Here's how the part is built. I have some questions about the finished solid (model axes, mm). A direction names the side the tool comes from. Round coordinates to 2 decimals unless told otherwise and drop trailing zeros. Write each loop counter-clockwise with the first axis right and the second up, starting at its lowest first coordinate (ties: lowest second). Pieces come first, ordered by that corner, then holes. Notation, with made-up numbers: (-34, 59) -> (-6, 59) arc R29 cw to (-6, 97) -> close; hole circle Ø5 at (19.5, 77.5). An arc over 180 degrees is marked (long way). Answer as CSV lines item,"result".
from build123d import *

# Parameters (mm, degrees)
EXTRUDE_1_DEPTH = 2
EXTRUDE_2_DEPTH = 1


with BuildPart() as part:
    # Эскиз1 → Бобышка-Вытянуть1 (new body)
    with BuildSketch(Plane.XY):
        with BuildLine():
            Line((-1.75, -2.25), (1.75, -2.25))
            ThreePointArc((1.75, -2.25), (2.457106781, -1.957106781), (2.75, -1.25))
            Line((2.75, -1.25), (2.75, 1.25))
            ThreePointArc((2.75, 1.25), (2.457106781, 1.957106781), (1.75, 2.25))
            Line((1.75, 2.25), (-1.75, 2.25))
            ThreePointArc((-1.75, 2.25), (-2.457106781, 1.957106781), (-2.75, 1.25))
            Line((-2.75, 1.25), (-2.75, -1.25))
            ThreePointArc((-2.75, -1.25), (-2.457106781, -1.957106781), (-1.75, -2.25))
        make_face()
    extrude(amount=EXTRUDE_1_DEPTH)

    # Эскиз2 → Бобышка-Вытянуть2 (add)
    with BuildSketch(Plane.XY.offset(2)):
        with BuildLine():
            Line((-3.25, -3.25), (3.25, -3.25))
            ThreePointArc((3.25, -3.25), (3.957106781, -2.957106781), (4.25, -2.25))
            Line((4.25, -2.25), (4.25, 2.25))
            ThreePointArc((4.25, 2.25), (3.957106781, 2.957106781), (3.25, 3.25))
            Line((3.25, 3.25), (-3.25, 3.25))
            ThreePointArc((-3.25, 3.25), (-3.957106781, 2.957106781), (-4.25, 2.25))
            Line((-4.25, 2.25), (-4.25, -2.25))
            ThreePointArc((-4.25, -2.25), (-3.957106781, -2.957106781), (-3.25, -3.25))
        make_face()
    extrude(amount=EXTRUDE_2_DEPTH)


solid = part.part
Item 1: For faces 1 (the cylindrical face through (2.465, 1.949, 0.986)), 2 (the cylindrical face through (-2.465, -1.949, 0.986)), 3 (the flat face through (0, 2.25, 1)), 4 (the cylindrical face through (-2.449, 1.965, 0.986)), 5 (the cylindrical face through (2.449, -1.965, 0.986)), which set-ups out of +Z, -Z, +X, -X, +Y, -Y let a thin tool reach every point of the face, with its end or its side?
Results found:
face 1,"-Z, +X, +Y"
face 2,"-Z, -X, -Y"
face 3,"-Z, +X, -X, +Y"
face 4,"-Z, -X, +Y"
face 5,"-Z, +X, -Y"
Item 2: I need wall thicknesses on L1, parallel to Z at x = -3, y = 1.25; L2, parallel to Y at x = 1, z = 1.8; L3, parallel to X at y = -0.75, z = 0.45. Which ranges of each line are inside material? Lowest first, please.
Results found:
L1,"z = 2 to 3"
L2,"y = -2.25 to 2.25"
L3,"x = -2.75 to 2.75"
Item 3: Suppose I cut it at C-C, the plane y = -2.5. List the corners of the cut face in (x, z) for me.
Results found:
outline,"(-4.22, 2) -> (4.22, 2) -> (4.22, 3) -> (-4.22, 3) -> close"
Item 4: Suppose I cut it at A-A, the plane x = 0.75. List the corners of the cut face in (y, z) for me.
Results found:
outline,"(-3.25, 2) -> (-2.25, 2) -> (-2.25, 0) -> (2.25, 0) -> (2.25, 2) -> (3.25, 2) -> (3.25, 3) -> (-3.25, 3) -> close"
Item 5: Suppose I cut it at B-B, the plane z = 0.85. List the corners of the cut face in (x, y) for me.
Results found:
outline,"(-2.75, -1.25) arc R1 ccw to (-1.75, -2.25) -> (1.75, -2.25) arc R1 ccw to (2.75, -1.25) -> (2.75, 1.25) arc R1 ccw to (1.75, 2.25) -> (-1.75, 2.25) arc R1 ccw to (-2.75, 1.25) -> close"
Item 6: Will these pins go through, and if not, where does the flat tip stop? pin 1 (1 mm diameter, centred on x = -0.5, z = 0.5, fed in from +Y); pin 2 (1.5 mm diameter, centred on x = 3, z = 0.5, fed in from +Y); pin 3 (0.6 mm diameter, centred on y = 0.5, z = 1.5, fed in from +X).
Results found:
pin 1,"stops at y = 2.25"
pin 2,"stops at y = 2.12"
pin 3,"stops at x = 2.75"
